Source: CAD feature listing. Evaluate the final solid. Frame: model axes, mm. Round coordinates to 2 decimals unless told otherwise and drop trailing zeros. Write each loop counter-clockwise with the first axis right and the second up, starting at its lowest first coordinate (ties: lowest second). Pieces come first, ordered by that corner, then holes. Notation, with made-up numbers: (61, 15) -> (109, 15) arc R29 cw to (109, 40) -> close; hole circle Ø11 at (45.25, 80). An arc over 180 degrees is marked (long way). Return JSON: item names as keys, results as strings. Group by question number.
from build123d import *

# Parameters (mm, degrees)
CROQUIS1_R              = 1.5
CROQUIS1_W              = 5
CROQUIS1_H              = 70
SALIENTE_EXTRUIR1_DEPTH = 5


with BuildPart() as part:
    # Croquis1 → Saliente-Extruir1 (new body)
    with BuildSketch(Plane.XY):
        Polygon((0, 0), (31, 0), (31, 15), (27.5, 15), (27.5, 18), (31, 18), (31, 21), (34, 21), (34, 18), (37.5, 18), (37.5, 15), (34, 15), (34, 0), (50, 0), (50, -10), (90, -10), (90, 0), (106, 0), (106, 15), (102.5, 15), (102.5, 18), (106, 18), (106, 21), (109, 21), (109, 18), (112.5, 18), (112.5, 15), (109, 15), (109, 0), (140, 0), (140, 210), (109, 210), (109, 195), (112.5, 195), (112.5, 192), (109, 192), (109, 189), (106, 189), (106, 192), (102.5, 192), (102.5, 195), (106, 195), (106, 210), (90, 210), (90, 215), (50, 215), (50, 210), (34, 210), (34, 195), (37.5, 195), (37.5, 192), (34, 192), (34, 189), (31, 189), (31, 192), (27.5, 192), (27.5, 195), (31, 195), (31, 210), (0, 210), align=None)
        with Locations((12.5, 175)):
            Circle(CROQUIS1_R, mode=Mode.SUBTRACT)
        with Locations(Location((12.5, 35, 0), (0, 0, 180))):
            Circle(CROQUIS1_R, mode=Mode.SUBTRACT)
        with Locations(Location((127.5, 175, 0), (0, 0, 180))):
            Circle(CROQUIS1_R, mode=Mode.SUBTRACT)
        with Locations((127.5, 35)):
            Circle(CROQUIS1_R, mode=Mode.SUBTRACT)
        with Locations((127.5, 105)):
            Rectangle(CROQUIS1_W, CROQUIS1_H, mode=Mode.SUBTRACT)
        with Locations((12.5, 105)):
            Rectangle(CROQUIS1_W, CROQUIS1_H, mode=Mode.SUBTRACT)
    extrude(amount=SALIENTE_EXTRUIR1_DEPTH)


solid = part.part
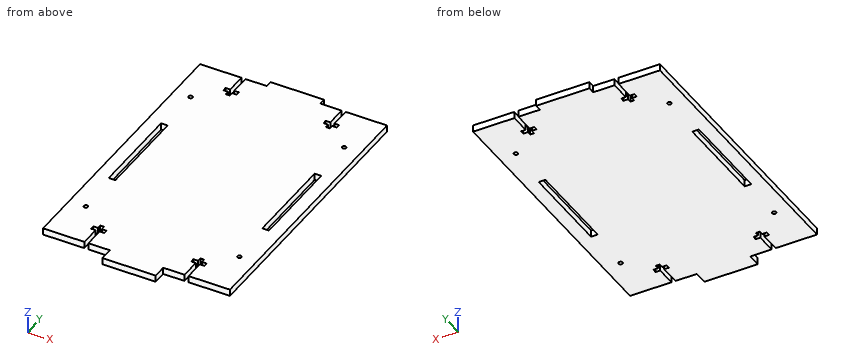
Item 1: Cut plane B-B on z = 1.8. Give the number of separate pieces and of enclosed holes in the cut face, and give its area (3 significant figures).
Item 2: Cut plane A-A on y = 125. Output: boundary loops of the cut face in (x, z).
Item 3: First-contact query: pin 1 Ø1.5 at (x, z) = (128.5, 3) entering from +Y; pin 2 Ø1 at (x, z) = (29.5, 3.5) entering from -Y. Flat tips, straight axial feed; report the tip coordinate or a pass-through.
Item 4: Material intervals for probe 1 along X at (y, z) = (175, 2.1); probe 2 along X at (y, z) = (131.5, 0.95); probe 3 along Y at (x, z) = (127.5, 3.15), sorted ascending.
Here are the results:
{
 "1": {"separate pieces": "1", "enclosed holes": "6", "area": "28,900 mm^2"},
 "2": {"outline": "(0, 0) -> (10, 0) -> (10, 5) -> (0, 5) -> close; (15, 0) -> (125, 0) -> (125, 5) -> (15, 5) -> close; (130, 0) -> (140, 0) -> (140, 5) -> (130, 5) -> close"},
 "3": {"pin 1": "stops at y = 210", "pin 2": "stops at y = 0"},
 "4": {"probe 1": "x = 0 to 11, 14 to 126, 129 to 140", "probe 2": "x = 0 to 10, 15 to 125, 130 to 140", "probe 3": "y = 0 to 33.5, 36.5 to 70, 140 to 173.5, 176.5 to 210"}
}
